Model file for the job. Use its own axes, mm. A direction names the side the tool comes from. Coordinates: 2 decimals unless noted, no trailing zeros. Loops run counter-clockwise (first coordinate to the right, second up) from the corner with the lowest first, then second, coordinate; pieces in that order, holes last.
Autodesk Inventor part; units mm, degrees
ref_plane "Work Plane1" through (0, 0, 5) normal (0, 0, 1) x (1, 0, 0)
ref_plane "YZ Plane" through (0, 0, 0) normal (1, 0, 0) x (0, 1, 0)
ref_plane "XZ Plane" through (0, 0, 0) normal (0, 1, 0) x (-1, 0, 0)
sketch "Sketch1" plane through (0, 0, 0) normal (0, 0, 1) x (1, 0, 0)
  line L0 (14.6962, 12.74) -> (14.6962, 0) construction
  line L1 (10.61, 12.2) -> (1.53, 12.2)
  arc A0 (1.53, 12.2) -> (0, 10.67) centre (1.53, 10.67) ccw
  line L2 (0, 10.67) -> (0, 1.53)
  arc A1 (0, 1.53) -> (1.53, 0) centre (1.53, 1.53) ccw
  line L3 (1.53, 0) -> (10.61, 0)
  arc A2 (10.61, 0) -> (12.14, 1.53) centre (10.61, 1.53) ccw
  arc A3 (12.14, 10.67) -> (10.61, 12.2) centre (10.61, 10.67) ccw
  line L4 (12.14, 10.67) -> (12.14, 1.53)
  point P0 (0, 0)
  point P1 (0, 0)
  dimension "d10" = 12.74
ref_plane "Work Plane1" through (0, 0, 5) normal (0, 0, 1) x (1, 0, 0)
sketch "Sketch2" plane through (0, 0, 5) normal (0, 0, 1) x (1, 0, 0)
  line L0 (10.88, 12.74) -> (1.8, 12.74)
  line L1 (10.88, 12.74) -> (1.8, 12.74)
  arc A0 (1.8, 12.74) -> (0, 10.94) centre (1.8, 10.94) ccw
  line L2 (0, 10.94) -> (0, 1.8)
  arc A1 (0, 1.8) -> (1.8, 0) centre (1.8, 1.8) ccw
  line L3 (1.8, 0) -> (10.88, 0)
  arc A2 (10.88, 0) -> (12.68, 1.8) centre (10.88, 1.8) ccw
  line L4 (12.68, 1.8) -> (12.68, 10.94)
  arc A3 (12.68, 10.94) -> (10.88, 12.74) centre (10.88, 10.94) ccw
  circle A4 centre (6.34, 6.37) radius 2.8
  line L5 (5.665, 8.395) -> (7.015, 8.395)
  line L6 (7.015, 4.345) -> (5.665, 4.345)
  line L7 (5.665, 4.345) -> (7.015, 8.395) construction
  line L8 (5.665, 8.395) -> (7.015, 4.345) construction
  line L9 (8.365, 5.695) -> (8.365, 7.045)
  line L10 (4.315, 7.045) -> (4.315, 5.695)
  line L11 (4.315, 5.695) -> (8.365, 7.045) construction
  line L12 (8.365, 5.695) -> (4.315, 7.045) construction
  line L13 (4.315, 5.695) -> (5.665, 5.695)
  line L14 (7.015, 5.695) -> (8.365, 5.695)
  line L15 (5.665, 4.345) -> (5.665, 5.695)
  line L16 (5.665, 7.045) -> (5.665, 8.395)
  line L17 (8.365, 7.045) -> (7.015, 7.045)
  line L18 (5.665, 7.045) -> (4.315, 7.045)
  line L19 (7.015, 8.395) -> (7.015, 7.045)
  line L20 (7.015, 5.695) -> (7.015, 4.345)
  point P0 (0, 0)
  dimension "d3" = 5.6
  dimension "d4" = 4.05
  dimension "d5" = 1.35
  dimension "d6" = 4.05
  dimension "d7" = 1.35
extrude "Extrusion3" add sketch "Sketch1" along normal blind 5
sketch "Sketch3" plane through (0, 0, 5) normal (0, 0, 1) x (1, 0, 0)
  line L0 (10.61, 12.47) -> (1.53, 12.47)
  line L1 (10.61, 12.47) -> (1.53, 12.47)
  arc A0 (1.53, 12.47) -> (-0.27, 10.67) centre (1.53, 10.67) ccw
  line L2 (-0.27, 10.67) -> (-0.27, 1.53)
  arc A1 (-0.27, 1.53) -> (1.53, -0.27) centre (1.53, 1.53) ccw
  line L3 (1.53, -0.27) -> (10.61, -0.27)
  arc A2 (10.61, -0.27) -> (12.41, 1.53) centre (10.61, 1.53) ccw
  line L4 (12.41, 1.53) -> (12.41, 10.67)
  arc A3 (12.41, 10.67) -> (10.61, 12.47) centre (10.61, 10.67) ccw
  circle A4 centre (6.07, 6.1) radius 2.8
  line L5 (5.395, 8.125) -> (6.745, 8.125)
  line L6 (6.745, 4.075) -> (5.395, 4.075)
  line L7 (5.395, 4.075) -> (6.745, 8.125) construction
  line L8 (5.395, 8.125) -> (6.745, 4.075) construction
  line L9 (8.095, 5.425) -> (8.095, 6.775)
  line L10 (4.045, 6.775) -> (4.045, 5.425)
  line L11 (4.045, 5.425) -> (8.095, 6.775) construction
  line L12 (8.095, 5.425) -> (4.045, 6.775) construction
  line L13 (4.045, 5.425) -> (5.395, 5.425)
  line L14 (6.745, 5.425) -> (8.095, 5.425)
  line L15 (5.395, 4.075) -> (5.395, 5.425)
  line L16 (5.395, 6.775) -> (5.395, 8.125)
  line L17 (8.095, 6.775) -> (6.745, 6.775)
  line L18 (5.395, 6.775) -> (4.045, 6.775)
  line L19 (6.745, 8.125) -> (6.745, 6.775)
  line L20 (6.745, 5.425) -> (6.745, 4.075)
  line L21 (10.61, 12.2) -> (1.53, 12.2)
  line L22 (0, 10.67) -> (0, 1.53)
  point P0 (0, 0)
  point P1 (-0.27, -0.27)
  point P2 (6.07, 12.2)
  point P3 (0, 6.1)
  point P4 (6.07, 6.1)
  dimension "d14" = 5.6
  dimension "d15" = 4.05
  dimension "d16" = 1.35
  dimension "d17" = 4.05
  dimension "d18" = 1.35
extrude "Extrusion4" add sketch "Sketch3" along normal blind 4.8 contours A4
sketch "Sketch4" plane through (0, 0, 0) normal (0, 0, -1) x (-1, 0, 0)
  line L0 (-1.53, 0) -> (-10.61, 0)
  line L1 (-7.4059, 5.3236) -> (-4.7341, 5.3236) construction
  line L2 (-4.7341, 5.3236) -> (-4.7341, 2.2661) construction
  line L3 (-4.7341, 2.2661) -> (-7.4059, 2.2661) construction
  line L4 (-7.4059, 2.2661) -> (-7.4059, 5.3236) construction
  line L5 (-11.8005, 9.9984) -> (-0.3395, 9.9984) construction
  line L6 (-0.3395, 9.9984) -> (-0.3395, 6.8396) construction
  line L7 (-0.3395, 6.8396) -> (-11.8005, 6.8396) construction
  line L8 (-11.8005, 6.8396) -> (-11.8005, 9.9984) construction
  line L9 (-10.8983, 6.894) -> (-10.8983, 9.3632)
  line L10 (-10.8983, 9.3632) -> (-11.8005, 9.3632)
  line L11 (-11.8005, 9.3632) -> (-11.8005, 9.944)
  line L12 (-11.8005, 9.944) -> (-9.23, 9.944)
  line L13 (-9.23, 9.944) -> (-9.23, 9.3632)
  line L14 (-9.23, 9.3632) -> (-10.1321, 9.3632)
  line L15 (-10.1321, 9.3632) -> (-10.1321, 6.894)
  line L16 (-10.1321, 6.894) -> (-10.8983, 6.894)
  line L17 (-7.6506, 7.9568) -> (-9.0075, 7.9568)
  line L18 (-9.0075, 7.9568) -> (-9.0075, 8.5253)
  line L19 (-9.0075, 8.5253) -> (-7.6506, 8.5253)
  line L20 (-7.6506, 8.5253) -> (-7.6506, 7.9568)
  line L21 (-5.5893, 6.894) -> (-7.2304, 6.894)
  line L22 (-7.2304, 6.894) -> (-7.2304, 7.4254)
  line L23 (-7.2304, 7.4254) -> (-6.793, 7.4254)
  line L24 (-6.793, 7.4254) -> (-6.793, 9.4126)
  line L25 (-6.793, 9.4126) -> (-7.2304, 9.4126)
  line L26 (-7.2304, 9.4126) -> (-7.2304, 9.944)
  line L27 (-7.2304, 9.944) -> (-5.5893, 9.944)
  line L28 (-5.5893, 9.944) -> (-5.5893, 9.4126)
  line L29 (-5.5893, 9.4126) -> (-6.0267, 9.4126)
  line L30 (-6.0267, 9.4126) -> (-6.0267, 7.4254)
  line L31 (-6.0267, 7.4254) -> (-5.5893, 7.4254)
  line L32 (-5.5893, 7.4254) -> (-5.5893, 6.894)
  line L33 (-3.046, 6.894) -> (-5.0801, 6.894)
  line L34 (-5.0801, 6.894) -> (-5.0801, 9.944)
  line L35 (-5.0801, 9.944) -> (-4.3139, 9.944)
  line L36 (-4.3139, 9.944) -> (-4.3139, 7.4748)
  line L37 (-4.3139, 7.4748) -> (-3.046, 7.4748)
  line L38 (-3.046, 7.4748) -> (-3.046, 6.894)
  spline S0 degree 2 poles (-1.7385, 6.8396) (-2.0894, 6.8396) (-2.6184, 6.9756) (-2.8457, 7.0744) knots 0 0 0 1 2 2 2
  line L39 (-2.8457, 7.0744) -> (-2.8457, 7.8011)
  line L40 (-2.8457, 7.8011) -> (-2.7765, 7.8011)
  spline S1 degree 2 poles (-2.7765, 7.8011) (-2.5467, 7.6058) (-1.9955, 7.3957) (-1.736, 7.3957) knots 0 0 0 1 2 2 2
  spline S2 degree 2 poles (-1.736, 7.3957) (-1.6692, 7.3957) (-1.4542, 7.4254) (-1.39, 7.4551) knots 0 0 0 1 2 2 2
  spline S3 degree 2 poles (-1.39, 7.4551) (-1.3109, 7.4897) (-1.1996, 7.6157) (-1.1996, 7.717) knots 0 0 0 1 2 2 2
  spline S4 degree 2 poles (-1.1996, 7.717) (-1.1996, 7.8332) (-1.3801, 7.9766) (-1.5037, 8.0087) knots 0 0 0 1 2 2 2
  spline S5 degree 2 poles (-1.5037, 8.0087) (-1.6594, 8.0507) (-2.0128, 8.1224) (-2.1685, 8.1768) knots 0 0 0 1 2 2 2
  spline S6 degree 2 poles (-2.1685, 8.1768) (-2.522, 8.3004) (-2.8284, 8.723) (-2.8284, 9.0394) knots 0 0 0 1 2 2 2
  spline S7 degree 2 poles (-2.8284, 9.0394) (-2.8284, 9.467) (-2.1043, 9.9984) (-1.5605, 9.9984) knots 0 0 0 1 2 2 2
  spline S8 degree 2 poles (-1.5605, 9.9984) (-1.2886, 9.9984) (-0.7498, 9.8871) (-0.5372, 9.7932) knots 0 0 0 1 2 2 2
  line L41 (-0.5372, 9.7932) -> (-0.5372, 9.0962)
  line L42 (-0.5372, 9.0962) -> (-0.604, 9.0962)
  spline S9 degree 2 poles (-0.604, 9.0962) (-0.7745, 9.242) (-1.2639, 9.4422) (-1.521, 9.4422) knots 0 0 0 1 2 2 2
  spline S10 degree 2 poles (-1.521, 9.4422) (-1.6223, 9.4422) (-1.7805, 9.4126) (-1.8695, 9.373) knots 0 0 0 1 2 2 2
  spline S11 degree 2 poles (-1.8695, 9.373) (-1.9411, 9.3409) (-2.0449, 9.2124) (-2.0449, 9.1333) knots 0 0 0 1 2 2 2
  spline S12 degree 2 poles (-2.0449, 9.1333) (-2.0449, 9.0147) (-1.8793, 8.8787) (-1.6421, 8.8243) knots 0 0 0 1 2 2 2
  spline S13 degree 2 poles (-1.6421, 8.8243) (-1.4888, 8.7897) (-1.2046, 8.723) (-1.0415, 8.6662) knots 0 0 0 1 2 2 2
  spline S14 degree 2 poles (-1.0415, 8.6662) (-0.7251, 8.55) (-0.4161, 8.1644) (-0.4161, 7.848) knots 0 0 0 1 2 2 2
  spline S15 degree 2 poles (-0.4161, 7.848) (-0.4161, 7.3933) (-1.1304, 6.8396) (-1.7385, 6.8396) knots 0 0 0 1 2 2 2
  line L43 (-4.9911, 2.2661) -> (-7.0055, 2.2661)
  line L44 (-7.0055, 2.2661) -> (-7.0055, 2.7975)
  line L45 (-7.0055, 2.7975) -> (-6.3629, 2.7975)
  line L46 (-6.3629, 2.7975) -> (-6.3629, 4.4115)
  line L47 (-6.3629, 4.4115) -> (-7.0055, 4.4115)
  line L48 (-7.0055, 4.4115) -> (-7.0055, 4.9083)
  spline S16 degree 2 poles (-7.0055, 4.9083) (-6.8646, 4.9083) (-6.5853, 4.9454) (-6.5013, 4.9849) knots 0 0 0 1 2 2 2
  spline S17 degree 2 poles (-6.5013, 4.9849) (-6.4049, 5.0344) (-6.2962, 5.2) (-6.2863, 5.3236) knots 0 0 0 1 2 2 2
  line L49 (-6.2863, 5.3236) -> (-5.6189, 5.3236)
  line L50 (-5.6189, 5.3236) -> (-5.6189, 2.7975)
  line L51 (-5.6189, 2.7975) -> (-4.9911, 2.7975)
  line L52 (-4.9911, 2.7975) -> (-4.9911, 2.2661)
  point P0 (0, 0)
  point P1 (-6.07, 0)
  point P2 (-6.07, 2.2661)
  point P3 (-6.07, 2.2661)
  point P4 (-6.07, 6.8396)
  point P5 (-6.07, 6.8396)
extrude "Extrusion5" add sketch "Sketch4" along normal blind 0.9
properties part number "IPC TILS 1 key"
Q1. Drill centre lines: line 1 (Z direction, x = 9.5, y = 4.5); line 2 (Y direction, x = 8, z = 8) (3 decimals); line 3 (Y direction, x = 5.25, z = 6.5) (3 decimals). Where is each one in solid material? Low to high.
Answers:
line 1: z = 0 to 5
line 2: y = 4.071 to 5.425, 6.775 to 8.129
line 3: y = 3.423 to 5.425, 6.775 to 8.777
Q2. Slice it at C-C (x = 4.5). List the corners of the cut face in (y, z) (3 decimals).
Answers:
outline: (0, 0) - (6.894, 0) - (6.894, -0.9) - (9.944, -0.9) - (9.944, 0) - (12.2, 0) - (12.2, 5) - (8.418, 5) - (8.418, 9.8) - (6.775, 9.8) - (6.775, 5) - (5.425, 5) - (5.425, 9.8) - (3.782, 9.8) - (3.782, 5) - (0, 5) - close
Q3. Slice it at A-A (y = 6.1). List the corners of the cut face in (x, z) (3 decimals).
Answers:
outline: (0, 0) - (12.14, 0) - (12.14, 5) - (8.87, 5) - (8.87, 9.8) - (8.095, 9.8) - (8.095, 5) - (4.045, 5) - (4.045, 9.8) - (3.27, 9.8) - (3.27, 5) - (0, 5) - close
Q4. Flat gauge pins, fed straight in: P1, Ø3, axis at x = 10, z = 5.5, coming from the -Y side; P2, Ø0.7, axis at y = 3.5, z = -0.5, coming from the +X side; P3, Ø2, axis at x = 6.5, y = 1.5, coming from the +Z side; P4, Ø0.5, axis at y = 8.5, z = -0.5, coming from the +X side. Where does each tip first touch, or does it go through?
Answers:
P1: stops at y = 0
P2: stops at x = 6.36
P3: stops at z = 5
P4: stops at x = 10.9
Q5. Slice it at B-B (z = 6.75). List the corners of the cut face in (x, y) (3 decimals), and give its area (3 significant figures).
Answers:
outline: circle Ø5.6 at (6.07, 6.1); hole (4.045, 5.425) - (5.395, 5.425) - (5.395, 4.075) - (6.745, 4.075) - (6.745, 5.425) - (8.095, 5.425) - (8.095, 6.775) - (6.745, 6.775) - (6.745, 8.125) - (5.395, 8.125) - (5.395, 6.775) - (4.045, 6.775) - close
area: 15.5 mm2
Q6. Which spindle directions (+Z, -Z, +X, -X, +Y, -Y) get a long thin tool onto all of the face, cutting with end or side? Do faces 1 (the flat face through (6, 2.266, -0.4)), 2 (the flat face through (5.08, 8.4, -0.4)), 3 (the flat face through (6.4, 9.944, -0.4)), 4 (the flat face through (5.395, 5, 7)), 5 (the flat face through (8.3, 7.957, -0.4)). Say none if no direction does.
Answers:
face 1: -Z, +X, -X, -Y
face 2: -Z, +Y
face 3: -Z, +X, +Y
face 4: +Z
face 5: -Z, -Y
Q7. Mould opens along X. For faces 6 (the cylindrical face through (5.463, 8.833, 7.366)), 7 (the flat face through (7, 5, 9.8)), 8 (the flat face through (5, 6.775, 7)) say: +X half, -X half, draft (parallel to the pull), parting line (faces both ways), or undercut.
Answers:
face 6: parting line
face 7: draft
face 8: undercut
Q8. Slice it at D-D (y = 3.5). List the corners of the cut face in (x, z).
Answers:
outline: (0, 0) - (5.62, 0) - (5.62, -0.9) - (6.36, -0.9) - (6.36, 0) - (12.14, 0) - (12.14, 5) - (7.11, 5) - (7.11, 9.8) - (5.03, 9.8) - (5.03, 5) - (0, 5) - close
